Could you check a few things on this model? Use its own coordinates, in mm. A direction names the side the tool comes from. Round coordinates to 2 decimals unless told otherwise and drop trailing zeros. Loops run counter-clockwise (first coordinate to the right, second up) from the corner with the lowest first, then second, coordinate; pieces in that order, holes last. Notation, with made-up numbers: M -34,65.5 L -16,65.5 A26 ccw -16,95.5 Z; hole C 64.5,71 d6. An arc over 180 degrees is marked long. Return JSON: item names as keys, results as strings. Group by question number.
```python
from build123d import *

# Parameters (mm, degrees)
F0_W      = 12.6
F0_H      = 32
F1_DEPTH  = 0.6
F2_W      = 15
F2_H      = 23
F3_DEPTH  = 0.66
F4_W      = 12.6
F4_H      = 7
F5_DEPTH  = 2.2
F6_W      = 12.6
F6_H      = 2
F7_DEPTH  = 2.2
F9_W      = 12.572133
F9_H      = 22.951454
F10_DEPTH = 1.54
F11_W     = 2.2
F11_H     = 9
F12_DEPTH = 4.5
F13_R     = 1
F14_DEPTH = 16
F15_R     = 3
F16_R     = 2
F17_R     = 3
F18_R     = 2


with BuildPart() as f1:
    # F0 (on Top) → F1 (new body)
    with BuildSketch(Plane.XY):
        with Locations((0.140124, -3.403742)):
            Rectangle(F0_W, F0_H)
    extrude(amount=F1_DEPTH)

    # F2 (on face) → F3 (join)
    with BuildSketch(Plane.XY.offset(0.6)):
        with Locations((0.070062, -0.903742)):
            Rectangle(F2_W, F2_H)
    extrude(amount=F3_DEPTH)

    # F4 (on face) → F5 (join)
    with BuildSketch(Plane.XY.offset(0.6)):
        with Locations((0.140124, -15.903742)):
            Rectangle(F4_W, F4_H)
    extrude(amount=F5_DEPTH)

    # F6 (on face) → F7 (join)
    with BuildSketch(Plane.XY.offset(0.6)):
        with Locations((0.140124, 11.596258)):
            Rectangle(F6_W, F6_H)
    extrude(amount=F7_DEPTH)

    # F9 (on face) → F10 (join)
    with BuildSketch(Plane.XY.offset(1.26)):
        with Locations((0.168414, -0.908688)):
            Rectangle(F9_W, F9_H)
    extrude(amount=F10_DEPTH)

    # F11 (on face) → F12 (join)
    with BuildSketch(Plane.XY.offset(2.8)):
        with Locations((-5.017652, -5.903742)):
            Rectangle(F11_W, F11_H)
        with Locations((5.354481, -5.903742)):
            Rectangle(F11_W, F11_H)
    extrude(amount=F12_DEPTH)

    # F13 (on face) → F14 (cut)
    with BuildSketch(Plane.YZ.offset(6.454481)):
        with Locations((-5.403742, 5)):
            Circle(F13_R)
    extrude(amount=-F14_DEPTH, mode=Mode.SUBTRACT)

    # F15
    f15_edges = [f1.edges().sort_by_distance(p)[0] for p in [
        (-5.017652, -10.403742, 7.3),
    ]]
    fillet(f15_edges, radius=F15_R)

    # F16
    f16_edges = [f1.edges().sort_by_distance(p)[0] for p in [
        (-5.017652, -1.403742, 7.3),
    ]]
    fillet(f16_edges, radius=F16_R)

    # F17
    f17_edges = [f1.edges().sort_by_distance(p)[0] for p in [
        (5.354481, -10.403742, 7.3),
    ]]
    fillet(f17_edges, radius=F17_R)

    # F18
    f18_edges = [f1.edges().sort_by_distance(p)[0] for p in [
        (5.354481, -1.403742, 7.3),
    ]]
    fillet(f18_edges, radius=F18_R)


solid = f1.part
```
1. If we section it at A-A, the plane z = 2.5: Please give me the cut outline in (x, y).
2. I need wall thicknesses on probe 1 along X at (y, z) = (-3.5, 5.5); probe 2 along Z at (x, y) = (-5.75, 1.5); probe 3 along X at (y, z) = (-11, 2.5). Which ranges of each line are inside material? Lowest first, please.
3. On a 3-axis mill with a long thin cutter (end or side, diameter ignored), from which of +Z, -Z, +X, -X, +Y, -Y can I reach the whole of each face in a straight line? I mean faces 4 (the face through (7, -1, 0.6)), 5 (the face through (-5, -1.404, 4)), 6 (the face through (-6.118, -6, 4)). Say none if no direction works.
4. We'd pull the mould along X, two halves only. Please class faces 1 (the face through (-6.118, -1, 2)), 2 (the face through (-3.918, -6, 4)), 3 (the face through (-5.002, -9.548, 6.398)): +X half, -X half, draft (parallel to the pull), parting line (faces both ways), or undercut.
5. If we section it at B-B, the plane y = 0: Please give me the cut outline in (x, z).
6. I'm going to push flat-ended pins straight in: pin 1 Ø1.5 at (x, y) = (-0.5, -3) entering from +Z; pin 2 Ø0.7 at (x, z) = (5, 4.5) entering from +Y; pin 3 Ø3.5 at (y, z) = (-6, 5.5) entering from +X; pin 4 Ø1.2 at (x, z) = (5.5, 3) entering from -Y. Where does each tip first touch, or does it pass through?
Geometry results:
{
 "1": {"outline": "M -6.16,-19.4 L 6.44,-19.4 L 6.44,-12.4 L -6.16,-12.4 Z; M -6.16,10.6 L 6.44,10.6 L 6.44,12.6 L -6.16,12.6 Z; M -6.12,-12.38 L 6.45,-12.38 L 6.45,10.57 L -6.12,10.57 Z"},
 "2": {"probe 1": "-6.12 to -3.92, 4.25 to 6.45", "probe 2": "0 to 2.8", "probe 3": "-6.12 to 6.45"},
 "3": {"face 4": "-Z, +X, +Y, -Y", "face 5": "+Z, +X, -X, +Y", "face 6": "+Z, -X, +Y, -Y"},
 "4": {"face 1": "-X half", "face 2": "undercut", "face 3": "draft"},
 "5": {"outline": "M -7.43,0.6 L -6.16,0.6 L -6.16,0 L 6.44,0 L 6.44,0.6 L 7.57,0.6 L 7.57,1.26 L 6.45,1.26 L 6.45,2.8 L -6.12,2.8 L -6.12,1.26 L -7.43,1.26 Z"},
 "6": {"pin 1": "z = 2.8", "pin 2": "y = -1.4", "pin 3": "x = 6.45", "pin 4": "y = -19.4"}
}
